from build123d import *

# Parameters (mm, degrees)
SKETCH1_W           = 330
SKETCH1_H           = 250
BOSS_EXTRUDE1_DEPTH = 6.9
SKETCH2_R           = 6
CUT_EXTRUDE1_DEPTH  = 7.9
SKETCH3_R           = 25
CUT_EXTRUDE2_DEPTH  = 7.9
SKETCH4_R           = 3
CUT_EXTRUDE3_DEPTH  = 7.9
FILLET1_R           = 20
SKETCH5_R           = 1.5
CUT_EXTRUDE4_DEPTH  = 7.9


with BuildPart() as part:
    # Sketch1 → Boss-Extrude1 (new body)
    with BuildSketch(Plane(origin=(0, 0, 0), x_dir=(1, 0, 0), z_dir=(0, 1, 0))):
        Rectangle(SKETCH1_W, SKETCH1_H)
    extrude(amount=BOSS_EXTRUDE1_DEPTH)

    # Sketch2 → Cut-Extrude1 (cut, through all)
    with BuildSketch(Plane(origin=(0, 6.9, 0), x_dir=(1, 0, 0), z_dir=(0, 1, 0))):
        with Locations((-145, 105)):
            Circle(SKETCH2_R)
        with Locations((145, 105)):
            Circle(SKETCH2_R)
        with Locations((145, -105)):
            Circle(SKETCH2_R)
        with Locations((-145, -105)):
            Circle(SKETCH2_R)
    extrude(amount=-CUT_EXTRUDE1_DEPTH, mode=Mode.SUBTRACT)

    # Sketch3 → Cut-Extrude2 (cut, through all)
    with BuildSketch(Plane(origin=(0, 6.9, 0), x_dir=(1, 0, 0), z_dir=(0, 1, 0))):
        Circle(SKETCH3_R)
    extrude(amount=-CUT_EXTRUDE2_DEPTH, mode=Mode.SUBTRACT)

    # Sketch4 → Cut-Extrude3 (cut, through all)
    with BuildSketch(Plane(origin=(0, 6.9, 0), x_dir=(1, 0, 0), z_dir=(0, 1, 0))):
        with Locations((-152.5, -62.5)):
            Circle(SKETCH4_R)
        with Locations((-102.5, -112.5)):
            Circle(SKETCH4_R)
        with Locations((-102.5, 112.5)):
            Circle(SKETCH4_R)
        with Locations((-152.5, 62.5)):
            Circle(SKETCH4_R)
        with Locations((152.5, 62.5)):
            Circle(SKETCH4_R)
        with Locations((102.5, 112.5)):
            Circle(SKETCH4_R)
        with Locations((102.5, -112.5)):
            Circle(SKETCH4_R)
        with Locations((152.5, -62.5)):
            Circle(SKETCH4_R)
    extrude(amount=-CUT_EXTRUDE3_DEPTH, mode=Mode.SUBTRACT)

    # Fillet1
    fillet1_edges = [part.edges().sort_by_distance(p)[0] for p in [
        (-165, 3.45, -125),
        (165, 3.45, -125),
        (165, 3.45, 125),
        (-165, 3.45, 125),
    ]]
    fillet(fillet1_edges, radius=FILLET1_R)

    # Sketch5 → Cut-Extrude4 (cut, through all)
    with BuildSketch(Plane(origin=(0, 6.9, 0), x_dir=(1, 0, 0), z_dir=(0, 1, 0))):
        with Locations((-125, 16.275)):
            Circle(SKETCH5_R)
        with Locations((-76.74, 16.275)):
            Circle(SKETCH5_R)
        with Locations((-125, -66.275)):
            Circle(SKETCH5_R)
        with Locations((-76.74, -58.909)):
            Circle(SKETCH5_R)
    extrude(amount=-CUT_EXTRUDE4_DEPTH, mode=Mode.SUBTRACT)


solid = part.part
Input: part model. Units: mm. Frame: model coordinates. Give positions to 0.01 mm unless a question says otherwise; leave off trailing zeros. Write each loop counter-clockwise with the first axis right and the second up, starting at its lowest first coordinate (ties: lowest second). Pieces come first, ordered by that corner, then holes. Notation, with made-up numbers: M -18,69.25 L 23,69.25 A12 cw 23,84.25 Z; hole C 7.5,6 d10. An arc over 180 degrees is marked long. Use one line per item in the form item = value.
1. Ray query, L1, parallel to Z at x = 145, y = 2.25; L2, parallel to X at y = 4, z = -62.5; L3, parallel to X at y = 2.75, z = 105. Return the intervals inside material, ascending.
Outcome:
L1 = -125 to -111, -99 to 99, 111 to 125
L2 = -165 to -155.5, -149.5 to 149.5, 155.5 to 165
L3 = -165 to -151, -139 to 139, 151 to 165
2. Cut plane A-A on z = 0. Return loops of the section in (x, y), and give its area (3 significant figures).
Outcome:
outline = M -165,0 L -25,0 L -25,6.9 L -165,6.9 Z; M 25,0 L 165,0 L 165,6.9 L 25,6.9 Z
area = 1,930 mm²
3. Cut plane B-B on y = 3.5. State how many separate pieces and enclosed holes the cut face has, and give its area (3 significant figures).
Outcome:
separate_pieces = 1
enclosed_holes = 17
area = 79,500 mm²
4. Mould query, pull axis X, two halves, no side actions, for faces 1 (the face through (-165, 3, 1)), 2 (the face through (158.986, 3.498, -119.297)), 3 (the face through (140.58, 3.5, 100.94)), 4 (the face through (-149.42, 3.5, 100.94)). Classes: released by +X, released by -X, zero draft, split by the parting line, or undercut.
Outcome:
face_1 = released by -X
face_2 = released by +X
face_3 = undercut
face_4 = undercut
5. Cut plane C-C on x = -16.5. Return loops of the section in (y, z).
Outcome:
outline = M 0,-125 L 6.9,-125 L 6.9,-18.78 L 0,-18.78 Z; M 0,18.78 L 6.9,18.78 L 6.9,125 L 0,125 Z
